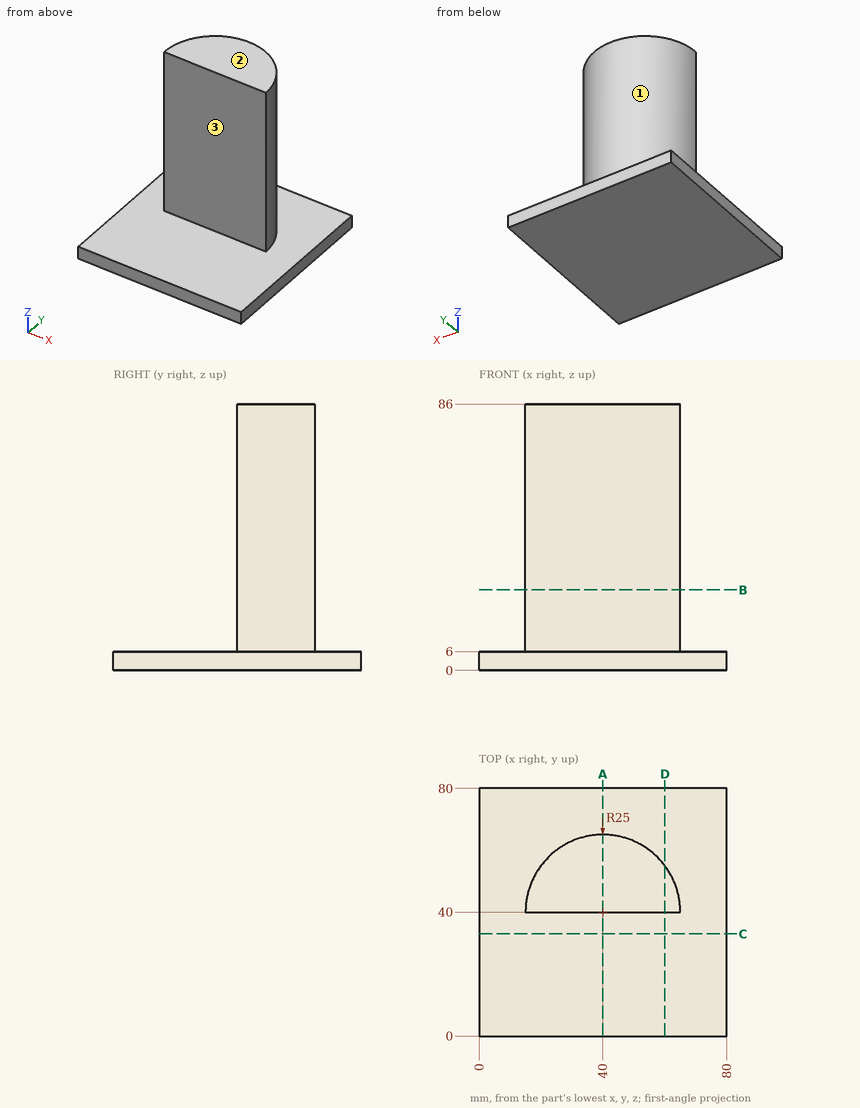
Geometry check sheet. Reference: drawing and pictorial views, mm from the part's lowest x, y, z. A direction names the side the tool comes from. Coordinates: 2 decimals unless noted, no trailing zeros. Loops run counter-clockwise (first coordinate to the right, second up) from the corner with the lowest first, then second, coordinate; pieces in that order, holes last. Notation, with made-up numbers: (37.25, -30) -> (74.25, -30) arc R29 cw to (74.25, -4) -> close; hole circle Ø9 at (82, 17). An arc over 180 degrees is marked (long way). Write item = value, one per line. Start each with the question number.
1. Tool access check on the marked faces 1, 2 and 3. Record the directions out of +Z, -Z, +X, -X, +Y, -Y that give a thin tool (end or side, any length) a straight path to the whole face; none if there is none.
2. Section check A-A on x = 40. Record the cut outline in (y, z), then the cut area to 3 significant figures.
3. Section check B-B on z = 26. Record the cut outline in (x, y), then the cut area to 3 significant figures.
4. Section check C-C on y = 33. Record the cut outline in (x, z), then the cut area to 3 significant figures.
5. Depth check by flat-ended pin: P1, Ø5, axis at x = 48, z = 29.5, coming from the +Y side; P2, Ø1.5, axis at x = 61.5, y = 19.5, coming from the +Z side; P3, Ø2, axis at x = 41, z = 20.5, coming from the -Y side. Enter the tip coordinate at first touch or a pass-through.
6. Section check D-D on x = 60. Record the cut outline in (y, z), then the cut area to 3 significant figures.
7. Material ranges on line 1 (Z direction, x = 69, y = 9); line 2 (X direction, y = 41, z = 82); line 3 (Y direction, x = 61.5, z = 15.5), recorded low to high.
Responses:
q1.face_1 = +Z, +Y
q1.face_2 = +Z, +X, -X, +Y, -Y
q1.face_3 = +Z, +X, -X, -Y
q2.outline = (0, 0) -> (80, 0) -> (80, 6) -> (65, 6) -> (65, 86) -> (40, 86) -> (40, 6) -> (0, 6) -> close
q2.area = 2,480 mm2
q3.outline = (15, 40) -> (65, 40) arc R25 ccw to start
q3.area = 982 mm2
q4.outline = (0, 0) -> (80, 0) -> (80, 6) -> (0, 6) -> close
q4.area = 480 mm2
q5.P1 = 64.39
q5.P2 = 6
q5.P3 = 40
q6.outline = (0, 0) -> (80, 0) -> (80, 6) -> (55, 6) -> (55, 86) -> (40, 86) -> (40, 6) -> (0, 6) -> close
q6.area = 1,680 mm2
q7.line_1 = 0 to 6
q7.line_2 = 15.02 to 64.98
q7.line_3 = 40 to 52.76
